from build123d import *

# Parameters (mm, degrees)
SKETCH1_W           = 40
SKETCH1_H           = 40
BOSS_EXTRUDE1_DEPTH = 5.6
SKETCH2_R           = 11
CUT_EXTRUDE1_DEPTH  = 6.6
SKETCH3_R           = 11.5
CUT_EXTRUDE2_DEPTH  = 7.5
SKETCH5_R           = 1.35
CUT_EXTRUDE4_DEPTH  = 6.6


with BuildPart() as part:
    # Sketch1 → Boss-Extrude1 (new body)
    with BuildSketch(Plane(origin=(0, 0, 0), x_dir=(1, 0, 0), z_dir=(0, 1, 0))):
        Rectangle(SKETCH1_W, SKETCH1_H)
    extrude(amount=BOSS_EXTRUDE1_DEPTH)

    # Sketch2 → Cut-Extrude1 (cut, through all)
    with BuildSketch(Plane(origin=(0, 5.6, 0), x_dir=(1, 0, 0), z_dir=(0, 1, 0))):
        Circle(SKETCH2_R)
    extrude(amount=-CUT_EXTRUDE1_DEPTH, mode=Mode.SUBTRACT)

    # Sketch3 → Cut-Extrude2 (cut)
    with BuildSketch(Plane(origin=(0, 0, 0), x_dir=(-1, 0, 0), z_dir=(0, -1, 0))):
        Circle(SKETCH3_R)
    extrude(amount=-CUT_EXTRUDE2_DEPTH, mode=Mode.SUBTRACT)

    # Sketch5 → Cut-Extrude4 (cut, through all)
    with BuildSketch(Plane(origin=(0, 5.6, 0), x_dir=(1, 0, 0), z_dir=(0, 1, 0))):
        with Locations((-15, 15)):
            Circle(SKETCH5_R)
        with Locations((15, 15)):
            Circle(SKETCH5_R)
        with Locations((15, -15)):
            Circle(SKETCH5_R)
        with Locations((-15, -15)):
            Circle(SKETCH5_R)
    extrude(amount=-CUT_EXTRUDE4_DEPTH, mode=Mode.SUBTRACT)


solid = part.part
For this review, take the finished solid that the model builds, in its own axes (mm). Give positions to 0.01 mm unless a question says otherwise; leave off trailing zeros. Order: outer loops, then holes, each group sorted by start corner. A loop starts at its lowest first (then second) coordinate and runs counter-clockwise, first axis right, second up. Notation, with made-up numbers: M 89,-13 L 101,-13 A21 ccw 101,4 Z; hole C 45.5,8 d9. An arc over 180 degrees is marked long. Answer in a Markdown table with one row per item. Add a question column.
(1) Consider section B-B on x = 0. State the section outline as (y, z) points, and give its area (3 significant figures).
(2) Wall thickness on probe 1 along Z at (x, y) = (15, 0.8); probe 2 along X at (y, z) = (1.2, -14): over which ranges is each line inside the solid? List them lowest first. Write a range as [from, to].
(3) Consider section C-C on y = 4.55. State the section outline as (x, z) points, and give its area (3 significant figures).
(4) Mouldability with a two-part tool opening along X and no side actions: class faces 1 (the face through (14.005, 2.839, -15.912)), 2 (the face through (20, 3, 0)), 3 (the face through (-20, 3, 0)) as +X half, -X half, draft (parallel to the pull), parting line (faces both ways), or undercut.
(5) Consider section A-A on z = 0. State the section outline as (x, y) points.
(6) Consider section D-D on x = -15. State the section outline as (y, z) points, and give its area (3 significant figures).
Evaluation:
| question | item | result |
|---|---|---|
| 1 | outline | M 0,-20 L 5.6,-20 L 5.6,-11.5 L 0,-11.5 Z; M 0,11.5 L 5.6,11.5 L 5.6,20 L 0,20 Z |
| 1 | area | 95.2 mm^2 |
| 2 | probe 1 | z = [-20, -16.35], [-13.65, 13.65], [16.35, 20] |
| 2 | probe 2 | x = [-20, -15.91], [-14.09, 14.09], [15.91, 20] |
| 3 | outline | M -20,-20 L 20,-20 L 20,20 L -20,20 Z; hole C -15,-15 d2.7; hole C -15,15 d2.7; hole C 0,0 d23; hole C 15,-15 d2.7; hole C 15,15 d2.7 |
| 3 | area | 1,160 mm^2 |
| 4 | face 1 | undercut |
| 4 | face 2 | +X half |
| 4 | face 3 | -X half |
| 5 | outline | M -20,0 L -11.5,0 L -11.5,5.6 L -20,5.6 Z; M 11.5,0 L 20,0 L 20,5.6 L 11.5,5.6 Z |
| 6 | outline | M 0,-20 L 5.6,-20 L 5.6,-16.35 L 0,-16.35 Z; M 0,-13.65 L 5.6,-13.65 L 5.6,13.65 L 0,13.65 Z; M 0,16.35 L 5.6,16.35 L 5.6,20 L 0,20 Z |
| 6 | area | 194 mm^2 |
